Autodesk Inventor part; units mm, degrees
ref_plane "YZ Plane" through (0, 0, 0) normal (1, 0, 0) x (0, 1, 0)
ref_plane "XZ Plane" through (0, 0, 0) normal (0, 1, 0) x (-1, 0, 0)
ref_plane "XY Plane" through (0, 0, 0) normal (0, 0, 1) x (1, 0, 0)
sketch "Sketch1" plane through (0, 0, 0) normal (0, 1, 0) x (-1, 0, 0)
  line L0 (0, 27.75) -> (3, 27.75)
  line L1 (3, 27.75) -> (3, 25.75)
  line L2 (-3, 25.75) -> (-3, 23.75)
  line L3 (8, 13.5) -> (8, 0)
  line L4 (-3, 26.75) -> (-3, 0)
  line L5 (8, 0) -> (0, 0)
  arc A0 (8, 13.5) -> (0, 23.75) centre (-2.5664, 13.5) ccw
  arc A1 (0, 25.75) -> (0, 23.75) centre (0, 24.75) ccw
  line L6 (0, 26.75) -> (-3, 26.75)
  line L7 (-3, 26.75) -> (-3, 25.75)
  line L8 (3, 25.75) -> (0, 25.75)
  line L9 (0, 27.75) -> (0, 26.75)
  line L10 (0, 0) -> (-3, 0)
  line L11 (8, 0) -> (8, 16.2)
  line L12 (8, 16.2) -> (10.5, 16.2)
  line L13 (10.5, 16.2) -> (10.5, 14.7)
  line L14 (10.5, 14.7) -> (10.5, 13.7)
  line L15 (10.5, 13.7) -> (10.5, 12.2)
  line L16 (10.5, 12.2) -> (8, 12.2)
  line L17 (10.5, 14.7) -> (12, 14.7)
  line L18 (12, 14.7) -> (12, 13.7)
  line L19 (12, 13.7) -> (10.5, 13.7)
  arc A2 (12, 14.7) -> (10.5, 16.2) centre (10.5, 14.7) ccw
  arc A3 (10.5, 12.2) -> (12, 13.7) centre (10.5, 13.7) ccw
  dimension "d0" = 27.75
  dimension "d7" = 13.5
  dimension "d8" = 11
  dimension "d9" = 10.5664
  dimension "d10" = 1
  dimension "d11" = 3
  dimension "d12" = 3
  dimension "d14" = 16.2
  dimension "d15" = 2.5
  dimension "d16" = 1.5
  dimension "d17" = 1
  dimension "d18" = 1.5
  dimension "d19" = 1.5
revolve "Revolution2" add sketch "Sketch1" angle 360 about axis through (-8, 0, 0) along (1, 0, 0)
properties part number "snow_can_top"
Input: part model. Units: mm. Frame: model coordinates. A direction names the side the tool comes from. Give positions to 0.01 mm unless a question says otherwise; leave off trailing zeros. Write each loop counter-clockwise with the first axis right and the second up, starting at its lowest first coordinate (ties: lowest second). Pieces come first, ordered by that corner, then holes. Notation, with made-up numbers: (12, -32.5) - (45, -32.5) arc R10 cw to (45, -24.5) - close; hole circle Ø9 at (10, -13.5). An arc over 180 degrees is marked (long way). Write item = value, one per line. Start each with the question number.
1) Draft query along Y for faces 4 (the face through (1.521, 26.114, -5.799)), 5 (the face through (-9.23, -0.54, -12.19)), 6 (the face through (-3, 25, 8)), 7 (the face through (-1.48, 25.14, -5.58)). Return one class per face: pulls with the +Y half, pulls with the -Y half, needs draft (parallel to the pull), parting line crosses it, or undercut.
2) Cut plane C-C (x = -6.5). Return loops of the section in (y, z).
3) Reachability of faces 1 (the face through (3, 0, 0)), 2 (the face through (-8, 0, 0)), 3 (the face through (0, -15, -23)) from +Z, -Z, +X, -X, +Y, -Y: full face, straight path, thin tool, end or side. Return the list, or none.
4) Pin query (flat end, axial travel): pin 1 (1 mm diameter, centred on x = -9, y = -0.5, fed in from -Z); pin 2 (2 mm diameter, centred on x = -5.5, z = -18.5, fed in from +Y); pin 3 (4 mm diameter, centred on x = -2.5, y = 18, fed in from +Z). Return the tip coordinate at first contact, or that it passes through.
5) Material intervals for L1, parallel to Y at x = -9.5, z = 0; L2, parallel to Z at x = -1.9, y = 0; L3, parallel to Z at x = -1.4, y = 0, sorted ascending. Write a range as [from, to].
6) Cut plane A-A (y = 0). Return loops of the section in (x, z).
Answers follow:
q1.face_4 = parting line crosses it
q1.face_5 = undercut
q1.face_6 = needs draft
q1.face_7 = undercut
q2.outline = circle Ø37.85 at (0, 0)
q3.face_1 = +Z, -Z, +X, +Y, -Y
q3.face_2 = -X
q3.face_3 = +X
q4.pin_1 = -16.2
q4.pin_2 = 11.31
q4.pin_3 = 22.67
q5.L1 = [-16.2, -12.2], [12.2, 16.2]
q5.L2 = [-27.75, -25.75], [-23.08, 23.08], [25.75, 27.75]
q5.L3 = [-27.75, -25.75], [-23.29, 23.29], [25.75, 27.75]
q6.outline = (-12, -14.7) arc R1.5 ccw to (-10.5, -16.2) - (-8, -16.2) - (-8, -13.5) arc R10.57 ccw to (0, -23.75) arc R1 cw to (0, -25.75) - (-3, -25.75) - (-3, -27.75) - (0, -27.75) - (0, -26.75) - (3, -26.75) - (3, 26.75) - (0, 26.75) - (0, 27.75) - (-3, 27.75) - (-3, 25.75) - (0, 25.75) arc R1 cw to (0, 23.75) arc R10.57 ccw to (-8, 13.5) - (-8, 16.2) - (-10.5, 16.2) arc R1.5 ccw to (-12, 14.7) - (-12, 13.7) arc R1.5 ccw to (-10.5, 12.2) - (-8, 12.2) - (-8, -12.2) - (-10.5, -12.2) arc R1.5 ccw to (-12, -13.7) - close
